from build123d import *

# Parameters (mm, degrees)
ESTRUSIONE_ESTRUSIONE1_DEPTH  = 260
SCHIZZO2_R                    = 9.5
TAGLIO_ESTRUSIONE1_DEPTH      = 40
TAGLIO_ESTRUSIONE2_START      = -80
SCHIZZO3_R                    = 9.5
TAGLIO_ESTRUSIONE2_DEPTH      = 80
TAGLIO_ESTRUSIONE3_DEPTH      = 263.488094968
TAGLIO_ESTRUSIONE3_DEPTH_BACK = 263.488094968
SCHIZZO5_R                    = 6
TAGLIO_ESTRUSIONE4_DEPTH      = 80
TAGLIO_ESTRUSIONE5_START      = -40
TAGLIO_ESTRUSIONE5_DEPTH      = 40


with BuildPart() as part:
    # Schizzo1 → Estrusione-Estrusione1 (new body)
    with BuildSketch(Plane(origin=(0, 0, 0), x_dir=(1, 0, 0), z_dir=(0, 1, 0))):
        with BuildLine():
            Line((-5, 15), (5, 15))
            ThreePointArc((5, 15), (20, 0), (5, -15))
            Line((5, -15), (-5, -15))
            ThreePointArc((-5, -15), (-20, 0), (-5, 15))
        make_face()
    extrude(amount=ESTRUSIONE_ESTRUSIONE1_DEPTH)

    # Schizzo2 → Taglio-Estrusione1 (cut)
    with BuildSketch(Plane.XZ):
        with BuildLine():
            Line((-5, -15), (5, -15))
            ThreePointArc((5, -15), (20, 0), (5, 15))
            Line((5, 15), (-5, 15))
            ThreePointArc((-5, 15), (-20, 0), (-5, -15))
        make_face()
        with Locations(Location((0, 0, 0), (0, 0, 270))):
            Circle(SCHIZZO2_R, mode=Mode.SUBTRACT)
    extrude(amount=-TAGLIO_ESTRUSIONE1_DEPTH, mode=Mode.SUBTRACT)

    # Schizzo3 → Taglio-Estrusione2 (cut)
    with BuildSketch(Plane(origin=(0, 260, 0), x_dir=(1, 0, 0), z_dir=(0, 1, 0)).offset(TAGLIO_ESTRUSIONE2_START)):
        with BuildLine():
            Line((-5, -15), (5, -15))
            ThreePointArc((5, -15), (20, 0), (5, 15))
            Line((5, 15), (-5, 15))
            ThreePointArc((-5, 15), (-20, 0), (-5, -15))
        make_face()
        with Locations(Location((0, 0, 0), (0, 0, 90))):
            Circle(SCHIZZO3_R, mode=Mode.SUBTRACT)
    extrude(amount=TAGLIO_ESTRUSIONE2_DEPTH, mode=Mode.SUBTRACT)

    # Schizzo4 → Taglio-Estrusione3 (cut, two sides: drawn at the far end of the back side and taken through both)
    with BuildSketch(Plane(origin=(0, 0, 15), x_dir=(0, 0, 1), z_dir=(-1, 0, 0)).offset(-TAGLIO_ESTRUSIONE3_DEPTH_BACK)):
        with BuildLine():
            Line((-9, 135), (-9, 85))
            ThreePointArc((-9, 85), (-15, 79), (-21, 85))
            Line((-21, 85), (-21, 135))
            ThreePointArc((-21, 135), (-15, 141), (-9, 135))
        make_face()
    extrude(amount=TAGLIO_ESTRUSIONE3_DEPTH + TAGLIO_ESTRUSIONE3_DEPTH_BACK, mode=Mode.SUBTRACT)

    # Schizzo5 → Taglio-Estrusione4 (cut)
    with BuildSketch(Plane(origin=(0, 0, -15), x_dir=(-1, 0, 0), z_dir=(0, 0, -1))):
        with Locations(Location((0, 110, 0), (0, 0, 326.442690238))):
            Circle(SCHIZZO5_R)
    extrude(amount=-TAGLIO_ESTRUSIONE4_DEPTH, mode=Mode.SUBTRACT)

    # Schizzo6 → Taglio-Estrusione5 (cut)
    with BuildSketch(Plane(origin=(0, 260, 0), x_dir=(1, 0, 0), z_dir=(0, 1, 0)).offset(TAGLIO_ESTRUSIONE5_START)):
        with BuildLine():
            Line((-2, -9.287087811), (-2, -8.5))
            Line((-2, -8.5), (2, -8.5))
            Line((2, -8.5), (2, -9.287087811))
            ThreePointArc((2, -9.287087811), (0, -9.5), (-2, -9.287087811))
        make_face()
    extrude(amount=TAGLIO_ESTRUSIONE5_DEPTH, mode=Mode.SUBTRACT)


solid = part.part
Build history of the part. All positions in model axes, mm. A direction names the side the tool comes from. Give positions to 0.01 mm unless a question says otherwise; leave off trailing zeros. Order: outer loops, then holes, each group sorted by start corner. A loop starts at its lowest first (then second) coordinate and runs counter-clockwise, first axis right, second up. Notation, with made-up numbers: M 41,-14 L 98,-14 A23 cw 98,22 Z; hole C 31,-18.5 d8. An arc over 180 degrees is marked long. Use one line per item in the form item = value.
Q1. Slice it at A-A, the plane z = 0. Write the cut outline in (x, y), and give its area (3 significant figures).
Conclusion:
outline = M -20,40 L -9.5,40 L -9.5,0 L 9.5,0 L 9.5,40 L 20,40 L 20,79 L -20,79 Z; M -20,141 L 20,141 L 20,180 L 9.5,180 L 9.5,260 L -9.5,260 L -9.5,180 L -20,180 Z
area = 5,400 mm2
Q2. Pull direction Y, two halves, no side cores. Call faces 5 (the cylindrical face through (0.635, 104.034, 10.437)), 6 (the flat face through (0, 260, 0)), 7 (the cylindrical face through (0, 79, 0)), 8 (the flat face through (0, 73, -15)): released by +Y, released by -Y, zero draft, split by the parting line, or undercut.
Conclusion:
face_5 = undercut
face_6 = released by +Y
face_7 = undercut
face_8 = zero draft
Q3. Pin check, flat tips, straight feed: P1, Ø1.5, axis at y = 92, z = -8, coming from the -X side; P2, Ø1, axis at x = 8, z = -9, coming from the -Y side; P3, Ø10, axis at x = -12, y = 94, coming from the +Z side. Stop position of each tip, or through.
Conclusion:
P1 = -18.13
P2 = 40
P3 = 14.87
Q4. Wall check: probe 1 along Z at (x, y) = (-5.5, 90); probe 2 along Y at (x, z) = (0, 12); probe 3 along Y at (x, z) = (-0.5, 7). Give the ranges that are in metal, low to high.
Conclusion:
probe_1 = -14.99 to -6, 6 to 14.99
probe_2 = 40 to 104, 116 to 180
probe_3 = 0 to 104.02, 115.98 to 260
Q5. Slice it at B-B, the plane y = 110. Write the cut outline in (x, z).
Conclusion:
outline = M -18.75,-6 A15 ccw -6,-14.97 L -6,-6 Z; M -18.75,6 L -6,6 L -6,14.97 A15 ccw Z; M 6,-14.97 A15 ccw 18.75,-6 L 6,-6 Z; M 6,6 L 18.75,6 A15 ccw 6,14.97 Z
Q6. Which spindle directions (+Z, -Z, +X, -X, +Y, -Y) get a long thin tool onto all of the face, cutting with end or side? Do faces 1 (the flat face through (-9, 180, -4)), 2 (the flat face through (-9, 40, 4)), 3 (the flat face through (0, 240, 8.5)), 4 (the cylindrical face through (0, 141, 0)). Say none if no direction does.
Conclusion:
face_1 = +Y
face_2 = -Y
face_3 = +Z, +Y
face_4 = +X, -X
